Input: part model. Units: mm. Frame: model coordinates. Face numbers are marked on the shaded views. A direction names the side the tool comes from. Give positions to 0.01 mm unless a question says otherwise; leave off trailing zeros. Loops run counter-clockwise (first coordinate to the right, second up) from the corner with the lowest first, then second, coordinate; pieces in that order, holes last. Notation, with made-up numbers: (73.25, 42.5) - (132.25, 42.5) arc R17 ccw to (132.25, 55.5) - close; hole circle Ø5 at (21, 78.5). An arc over 180 degrees is marked (long way). Answer as a JSON object with one key per item and string values. Group by question number.
(1) Section query A-A (x = 62). Return loops of the section in (y, z).
(2) Material intervals for L1, parallel to X at y = 119, z = 23.55; L2, parallel to Y at x = 62.25, z = 23; L3, parallel to Y at x = 66.5, z = 25.5, sorted ascending.
(3) Mould query, pull axis X, two halves, no side actions, for the marked faces 5, 6 and 7. Classes: +X half, -X half, draft (parallel to the pull), parting line (faces both ways), or undercut.
(4) Pin query (flat end, axial travel): P1, Ø4, axis at y = 106, z = 23, coming from the +X side; P2, Ø1.2, axis at y = 74.5, z = 23.5, coming from the -X side; P3, Ø6, axis at x = 63, y = 112.5, coming from the -Z side. Return the tip coordinate at first contact, or that it passes through.
(5) Section query B-B (y = 89). Return loops of the section in (x, z).
(6) Section query D-D (x = 58.5). Return loops of the section in (y, z).
(7) Access query for the marked faces 1, 2, 3 and 4. Directions: +Z, -Z, +X, -X, +Y, -Y. A direction counts if a zero-diameter tool reaches every point of the face in a straight line with its end or side. Return the directions, or none.
(8) Section query C-C (z = 24.5). Return loops of the section in (x, y).
```python
from build123d import *

# Parameters (mm, degrees)
SKETCH036_R             = 4.25
PAD014_DEPTH            = 4
SKETCH087_R             = 6
PAD030_DEPTH            = 10
SKETCH088_R             = 4.25
POCKET039_DEPTH         = 10
BODY005_PLACEMENT_ANGLE = 90


with BuildPart() as part:
    # Sketch036 → Pad014 (new body)
    with BuildSketch(Plane.XY):
        with BuildLine():
            ThreePointArc((5.67, 1.962422), (-6, 0), (5.67, -1.962422))
            Line((54.33, -1.962422), (5.67, -1.962422))
            ThreePointArc((54.33, -1.962422), (66, 0), (54.33, 1.962422))
            Line((5.67, 1.962422), (54.33, 1.962422))
        make_face()
        Circle(SKETCH036_R, mode=Mode.SUBTRACT)
        with Locations((60, 0)):
            Circle(SKETCH036_R, mode=Mode.SUBTRACT)
    extrude(amount=PAD014_DEPTH)

    # Sketch087 (on Face8 of Pad014) → Pad030 (join)
    with BuildSketch(Plane.XY.offset(4)):
        with Locations((30, 0)):
            Circle(SKETCH087_R)
    extrude(amount=-PAD030_DEPTH)

    # Sketch088 (on Face14 of Pad030) → Pocket039 (cut)
    with BuildSketch(Plane(origin=(0, 0, -6), x_dir=(1, 0, 0), z_dir=(0, 0, -1))):
        with Locations((30, 0)):
            Circle(SKETCH088_R)
    extrude(amount=-POCKET039_DEPTH, mode=Mode.SUBTRACT)


with BuildPart() as part_1:
    # Body005 placement: moved
    add(part.part.moved(Location((62, 59, 22))).rotate(Axis((62, 59, 22), (0, 0, 1)), BODY005_PLACEMENT_ANGLE))


solid = part_1.part
```
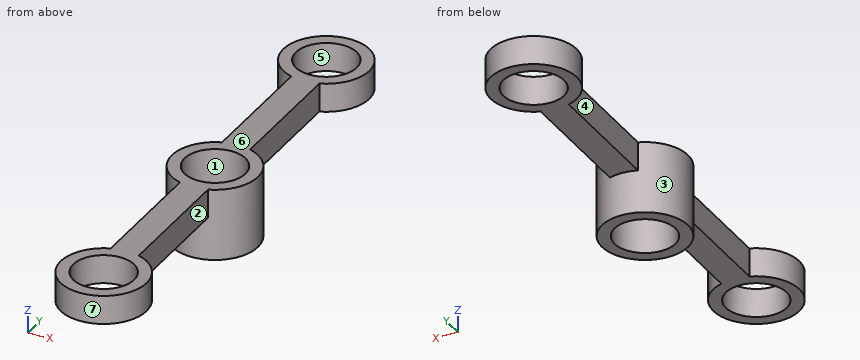
Recorded:
{
 "1": {"outline": "(53, 22) - (54.75, 22) - (54.75, 26) - (53, 26) - close; (63.25, 22) - (83, 22) - (83, 16) - (84.75, 16) - (84.75, 26) - (63.25, 26) - close; (93.25, 16) - (95, 16) - (95, 22) - (114.75, 22) - (114.75, 26) - (93.25, 26) - close; (123.25, 22) - (125, 22) - (125, 26) - (123.25, 26) - close"},
 "2": {"L1": "x = 56 to 57.75, 66.25 to 68", "L2": "y = 53.01 to 54.76, 63.24 to 84.76, 93.24 to 114.76, 123.24 to 124.99", "L3": "y = 55.03 to 62.97, 85.03 to 92.97, 115.03 to 122.97"},
 "3": {"face 5": "undercut", "face 6": "draft", "face 7": "parting line"},
 "4": {"P1": "stops at x = 63.96", "P2": "stops at x = 60.04", "P3": "stops at z = 22"},
 "5": {"outline": "(56, 16) - (57.75, 16) - (57.75, 26) - (56, 26) - close; (66.25, 16) - (68, 16) - (68, 26) - (66.25, 26) - close"},
 "6": {"outline": "(54.13, 22) - (56.59, 22) - (56.59, 26) - (54.13, 26) - close; (61.41, 22) - (63.87, 22) - (63.87, 26) - (61.41, 26) - close; (84.13, 16) - (86.59, 16) - (86.59, 26) - (84.13, 26) - close; (91.41, 16) - (93.87, 16) - (93.87, 26) - (91.41, 26) - close; (114.13, 22) - (116.59, 22) - (116.59, 26) - (114.13, 26) - close; (121.41, 22) - (123.87, 22) - (123.87, 26) - (121.41, 26) - close"},
 "7": {"face 1": "+Z, -Z", "face 2": "+Z, -Z, +X", "face 3": "-Z", "face 4": "+Z, -Z, -X"},
 "8": {"outline": "(60.04, 64.67) arc R6 ccw (long way) to (63.96, 64.67) - (63.96, 83.33) arc R6 ccw to (63.96, 94.67) - (63.96, 113.33) arc R6 ccw (long way) to (60.04, 113.33) - (60.04, 94.67) arc R6 ccw to (60.04, 83.33) - close; hole circle Ø8.5 at (62, 59); hole circle Ø8.5 at (62, 89); hole circle Ø8.5 at (62, 119)"}
}
